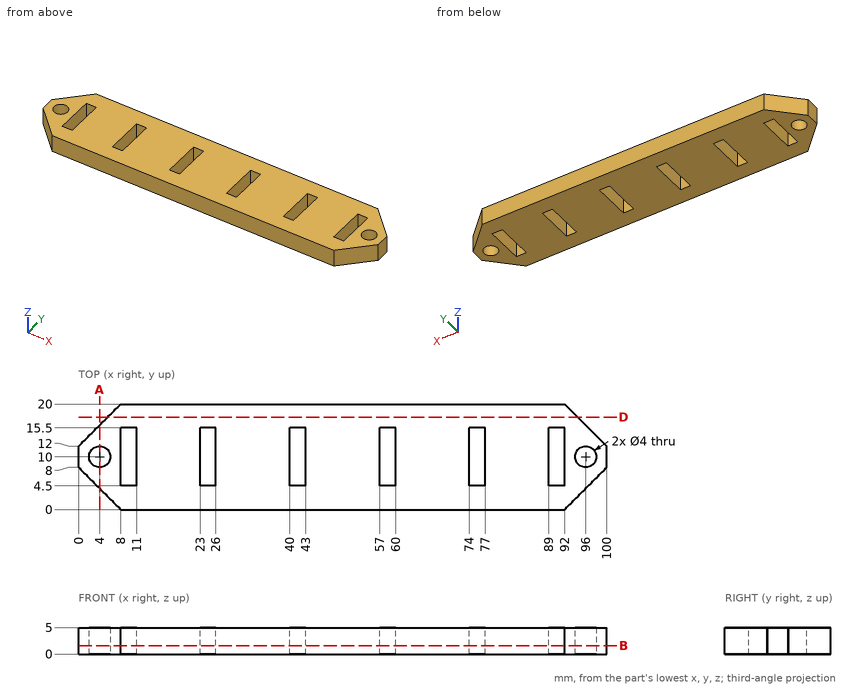
Geometry: see drawing. Coordinates: mm, zero at the bounding-box minimum. Round coordinates to 2 decimals unless told otherwise and drop trailing zeros. Loops run counter-clockwise (first coordinate to the right, second up) from the corner with the lowest first, then second, coordinate; pieces in that order, holes last. Notation, with made-up numbers: (5, -36.75) -> (43, -36.75) arc R21 ccw to (43, -0.75) -> close; hole circle Ø9 at (-11, 1.25). An arc over 180 degrees is marked (long way). One line per question, with ' | ' between items. Start each with the question number.
1. Contact query for a flat-ended pin moving along its axis: pin 1 (2.5 mm diameter, centred on x = 4, y = 10, fed in from -Z). Output: stop coordinate, or through.
2. Section B-B on z = 1.6. Count the separate pieces of the cut face and the enclosed holes in it, and give its area (3 significant figures).
3. Section A-A on x = 4. Output: boundary loops of the cut face in (y, z), and give its area (3 significant figures).
4. Section D-D on y = 17.5. Output: boundary loops of the cut face in (x, z), and give its area (3 significant figures).
5. Line query: line 1 along Y through (x, z) = (96, 2.7); line 2 along X through (y, z) = (18.5, 1.7); line 3 along Y through (x, z) = (7.5, 0.7). Output: solid intervals per line, ascending. Write a range as [from, to].
Returned:
1) pin 1: passes through
2) separate pieces: 1 | enclosed holes: 8 | area: 1,650 mm2
3) outline: (4, 0) -> (8, 0) -> (8, 5) -> (4, 5) -> close; (12, 0) -> (16, 0) -> (16, 5) -> (12, 5) -> close | area: 40.0 mm2
4) outline: (5.5, 0) -> (94.5, 0) -> (94.5, 5) -> (5.5, 5) -> close | area: 445 mm2
5) line 1: y = [4, 8], [12, 16] | line 2: x = [6.5, 93.5] | line 3: y = [0.5, 19.5]
